```python
from build123d import *

# Parameters (mm, degrees)
F0_R      = 2.5
F1_DEPTH  = 5
F2_W      = 5
F2_H      = 20
F3_DEPTH  = 15
F4_DEPTH  = 15
F5_R      = 10
F5_R_2    = 3
F6_DEPTH  = 5
F7_DEPTH  = 5
F8_R      = 10
F8_R_2    = 3
F9_DEPTH  = 5
F10_DEPTH = 5
F11_R     = 1
F12_R     = 1


with BuildPart() as f1:
    # F0 (on Top) → F1 (new body)
    with BuildSketch(Plane.XY):
        with BuildLine():
            ThreePointArc((-10.5, 0), (-14.8933982822, -10.6066017178), (-25.5, -15))
            Line((-25.5, -15), (25.5, -15))
            ThreePointArc((25.5, -15), (10.5, 0), (25.5, 15))
            Line((25.5, 15), (-25.5, 15))
            ThreePointArc((-25.5, 15), (-14.8933982822, 10.6066017178), (-10.5, 0))
        make_face()
        Circle(F0_R, mode=Mode.SUBTRACT)
        with BuildLine():
            ThreePointArc((-25.5, 15), (-40.5, 0), (-25.5, -15))
            Line((-25.5, -15), (-25.5, -2.5))
            ThreePointArc((-25.5, -2.5), (-28, 0), (-25.5, 2.5))
            Line((-25.5, 2.5), (-25.5, 15))
        make_face()
        with BuildLine():
            Line((-25.5, -2.5), (-25.5, -15))
            ThreePointArc((-25.5, -15), (-14.8933982822, -10.6066017178), (-10.5, 0))
            ThreePointArc((-10.5, 0), (-14.8933982822, 10.6066017178), (-25.5, 15))
            Line((-25.5, 15), (-25.5, 2.5))
            ThreePointArc((-25.5, 2.5), (-23.732233047, 1.767766953), (-23, 0))
            ThreePointArc((-23, 0), (-23.732233047, -1.767766953), (-25.5, -2.5))
        make_face()
        with BuildLine():
            ThreePointArc((25.5, 15), (10.5, 0), (25.5, -15))
            Line((25.5, -15), (25.5, -2.5))
            ThreePointArc((25.5, -2.5), (23, 0), (25.5, 2.5))
            Line((25.5, 2.5), (25.5, 15))
        make_face()
        with BuildLine():
            Line((25.5, -2.5), (25.5, -15))
            ThreePointArc((25.5, -15), (36.1066017178, -10.6066017178), (40.5, 0))
            ThreePointArc((40.5, 0), (36.1066017178, 10.6066017178), (25.5, 15))
            Line((25.5, 15), (25.5, 2.5))
            ThreePointArc((25.5, 2.5), (27.267766953, 1.767766953), (28, 0))
            ThreePointArc((28, 0), (27.267766953, -1.767766953), (25.5, -2.5))
        make_face()
    extrude(amount=F1_DEPTH)

    # F2 (on face) → F3 (join)
    with BuildSketch(Plane.XY.offset(5)):
        with Locations((13, 0)):
            Rectangle(F2_W, F2_H)
    extrude(amount=F3_DEPTH)

    # F2 (on face) → F4 (join)
    with BuildSketch(Plane.XY.offset(5)):
        with Locations((-13, 0)):
            Rectangle(F2_W, F2_H)
    extrude(amount=F4_DEPTH)

    # F5 (on face) → F6 (join)
    with BuildSketch(Plane.YZ.offset(-10.5)):
        with Locations((0, 20)):
            Circle(F5_R)
        with Locations((0, 20)):
            Circle(F5_R_2, mode=Mode.SUBTRACT)
    extrude(amount=-F6_DEPTH)

    # F5 (on face) → F7 (cut)
    with BuildSketch(Plane.YZ.offset(-10.5)):
        with BuildLine():
            ThreePointArc((-3, 20), (0, 17), (3, 20))
            Line((3, 20), (-3, 20))
        make_face()
    extrude(amount=-F7_DEPTH, mode=Mode.SUBTRACT)

    # F8 (on face) → F9 (join)
    with BuildSketch(Plane.YZ.offset(15.5)):
        with Locations((0, 20)):
            Circle(F8_R)
        with Locations((0, 20)):
            Circle(F8_R_2, mode=Mode.SUBTRACT)
    extrude(amount=-F9_DEPTH)

    # F8 (on face) → F10 (cut)
    with BuildSketch(Plane.YZ.offset(15.5)):
        with BuildLine():
            ThreePointArc((-3, 20), (0, 17), (3, 20))
            Line((3, 20), (-3, 20))
        make_face()
    extrude(amount=-F10_DEPTH, mode=Mode.SUBTRACT)

    # F11
    f11_edges = [f1.edges().sort_by_distance(p)[0] for p in [
        (-10.5, -10, 12.5),
        (15.5, -10, 12.5),
        (-15.5, -10, 12.5),
        (10.5, -10, 12.5),
    ]]
    fillet(f11_edges, radius=F11_R)

    # F12
    f12_edges = [f1.edges().sort_by_distance(p)[0] for p in [
        (0, -15, 5),
    ]]
    fillet(f12_edges, radius=F12_R)


solid = f1.part
```
CAD build for the part. Positions are in the model's coordinates, mm. A direction names the side the tool comes from. Round coordinates to 2 decimals unless told otherwise and drop trailing zeros. Write each loop counter-clockwise with the first axis right and the second up, starting at its lowest first coordinate (ties: lowest second). Pieces come first, ordered by that corner, then holes.
Item 1: Band-saw the part on A-A on z = 16. Write the cut outline in (x, y), then the cut area to 3 significant figures.
Filled in:
outline: (-15.5, -9) arc R1 ccw to (-14.5, -10) - (-11.5, -10) arc R1 ccw to (-10.5, -9) - (-10.5, 9) arc R1 ccw to (-11.5, 10) - (-14.5, 10) arc R1 ccw to (-15.5, 9) - close; (10.5, -9) arc R1 ccw to (11.5, -10) - (14.5, -10) arc R1 ccw to (15.5, -9) - (15.5, 9) arc R1 ccw to (14.5, 10) - (11.5, 10) arc R1 ccw to (10.5, 9) - close
area: 198 mm2
Item 2: Tool access for faces 1 (the flat face through (-15.5, -0.1, 16.8)), 2 (the flat face through (15.5, -0.1, 16.8)), 3 (the flat face through (-10.5, -0.1, 16.8)): list every direction of +Z, -Z, +X, -X, +Y, -Y with a clear straight run to the whole face (end or side of a thin tool).
Filled in:
face 1: +Z, -X, +Y, -Y
face 2: +Z, +X, +Y, -Y
face 3: +Z, +Y, -Y
Item 3: Mould opens along Y. For faces 4 (the flat face through (13, -10, 12)), 5 (the flat face through (13, 10, 12)), 6 (the flat face through (10.5, -0.1, 16.8)), 7 (the cylindrical face through (-12.96, 0.65, 22.93)) say: released by +Y, released by -Y, zero draft, split by the parting line, or undercut.
Filled in:
face 4: released by -Y
face 5: released by +Y
face 6: zero draft
face 7: undercut
Item 4: Drill centre lines: L1, parallel to X at y = 9, z = 18.5; L2, parallel to Z at x = -13.7, y = 0; L3, parallel to Y at x = 0, z = 1. Where is each one in solid material? Low to high.
Filled in:
L1: x = -15.5 to -10.5, 10.5 to 15.5
L2: z = 0 to 17, 23 to 30
L3: y = -15 to -2.5, 2.5 to 15
Item 5: Drop flat-ended pins along their axis: pin 1 Ø9 at (y, z) = (-2, 19.5) entering from -X; pin 2 Ø10 at (y, z) = (7, 23.5) entering from +X; pin 3 Ø1.5 at (x, z) = (13, 11) entering from +Y; pin 4 Ø12 at (x, y) = (-16.5, 8.5) entering from -Z. Give the stop position or say it passes through.
Filled in:
pin 1: stops at x = -15.5
pin 2: stops at x = 15.5
pin 3: stops at y = 10
pin 4: stops at z = 0
Item 6: Band-saw the part on B-B on x = 0. Write the cut outline in (y, z).
Filled in:
outline: (-15, 0) - (-2.5, 0) - (-2.5, 5) - (-14, 5) arc R1 ccw to (-15, 4) - close; (2.5, 0) - (15, 0) - (15, 4) arc R1 ccw to (14, 5) - (2.5, 5) - close
